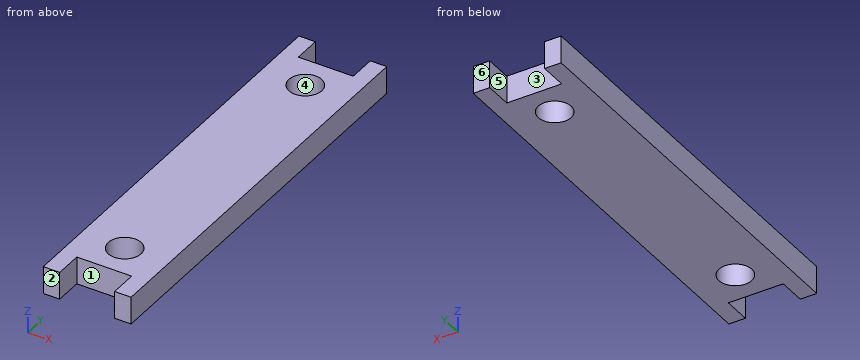
```python
from build123d import *

# Parameters (mm, degrees)
SKETCH2_R           = 3
BOSS_EXTRUDE1_DEPTH = 5


with BuildPart() as part:
    # Sketch2 → Boss-Extrude1 (new body)
    with BuildSketch(Plane.XY):
        Polygon((-5, 37.5), (-8, 37.5), (-8, -37.5), (-5, -37.5), (-5, -32.5), (5, -32.5), (5, -37.5), (8, -37.5), (8, 37.5), (5, 37.5), (5, 32.5), (-5, 32.5), align=None)
        with Locations(Location((0, -26.5, 0), (0, 0, 180))):
            Circle(SKETCH2_R, mode=Mode.SUBTRACT)
        with Locations((0, 26.5)):
            Circle(SKETCH2_R, mode=Mode.SUBTRACT)
    extrude(amount=BOSS_EXTRUDE1_DEPTH)


solid = part.part
```
Geometry check sheet. Reference: the model listing, model coordinates, mm. Face numbers are marked on the shaded views. A direction names the side the tool comes from. Coordinates: 2 decimals unless noted, no trailing zeros. Loops run counter-clockwise (first coordinate to the right, second up) from the corner with the lowest first, then second, coordinate; pieces in that order, holes last. Notation, with made-up numbers: (43, 5) - (69, 5) arc R13 ccw to (69, 13) - close; hole circle Ø6 at (38.25, 46.5). An arc over 180 degrees is marked (long way). One line per item, written item: value. Start each with the question number.
(1) Depth check by flat-ended pin: P1, Ø2.5, axis at x = -1.5, z = 2.5, coming from the -Y side. Enter the tip coordinate at first touch or a pass-through.
(2) Mould release check, pull along Y, two halves, no side actions. Record for the marked faces 4, 5 and 6: released by +Y, released by -Y, zero draft, split by the parting line, or undercut.
(3) Cross-section at B-B on z = 2.8. Enter the section's corners in (x, y), plus the area to 3 significant figures.
(4) Tool access check on the marked faces 1, 2 and 3. Record the directions out of +Z, -Z, +X, -X, +Y, -Y that give a thin tool (end or side, any length) a straight path to the whole face; none if there is none.
(5) Cross-section at D-D on x = -4.25. Enter the section's corners in (y, z), plus the area to 3 significant figures.
(6) Cross-section at C-C on x = 0. Enter the section's corners in (y, z).
(7) Material ranges on line 1 (Y direction, x = 0, z = 1.5); line 2 (Y direction, x = -3.25, z = 3.35); line 3 (Y direction, x = -1.5, z = 2.55), recorded low to high. Write a range as [from, to].
(8) Cross-section at A-A on y = -26.5. Enter the section's corners in (x, z).
Results below:
1. P1: stops at y = -32.5
2. face 4: undercut
2. face 5: zero draft
2. face 6: released by +Y
3. outline: (-8, -37.5) - (-5, -37.5) - (-5, -32.5) - (5, -32.5) - (5, -37.5) - (8, -37.5) - (8, 37.5) - (5, 37.5) - (5, 32.5) - (-5, 32.5) - (-5, 37.5) - (-8, 37.5) - close; hole circle Ø6 at (0, -26.5); hole circle Ø6 at (0, 26.5)
3. area: 1,040 mm2
4. face 1: +Z, -Z, -Y
4. face 2: +Z, -Z, +X, -X, -Y
4. face 3: +Z, -Z, +Y
5. outline: (-32.5, 0) - (32.5, 0) - (32.5, 5) - (-32.5, 5) - close
5. area: 325 mm2
6. outline: (-32.5, 0) - (-29.5, 0) - (-29.5, 5) - (-32.5, 5) - close; (-23.5, 0) - (23.5, 0) - (23.5, 5) - (-23.5, 5) - close; (29.5, 0) - (32.5, 0) - (32.5, 5) - (29.5, 5) - close
7. line 1: y = [-32.5, -29.5], [-23.5, 23.5], [29.5, 32.5]
7. line 2: y = [-32.5, 32.5]
7. line 3: y = [-32.5, -29.1], [-23.9, 23.9], [29.1, 32.5]
8. outline: (-8, 0) - (-3, 0) - (-3, 5) - (-8, 5) - close; (3, 0) - (8, 0) - (8, 5) - (3, 5) - close
